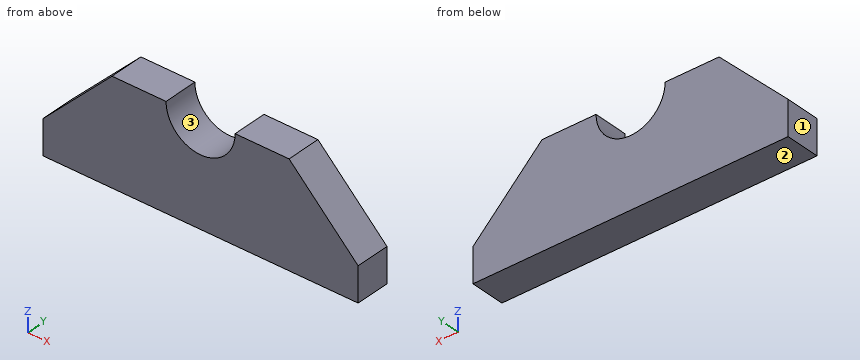
from build123d import *

# Parameters (mm, degrees)
F0_W     = 231.775
F0_H     = 25.4
F1_DEPTH = 76.2
F2_SIZE  = 50.8
F4_DEPTH = 25.4


with BuildPart() as f1:
    # F0 (on Top) → F1 (new body)
    with BuildSketch(Plane.XY):
        with Locations((-99.620111, 22.224578)):
            Rectangle(F0_W, F0_H)
    extrude(amount=F1_DEPTH)

    # F2
    f2_edges = [f1.edges().sort_by_distance(p)[0] for p in [
        (-215.507611, 22.224578, 76.2),
        (16.267389, 22.224578, 76.2),
    ]]
    chamfer(f2_edges, length=F2_SIZE)

    # F3 (on face) → F4 (cut)
    with BuildSketch(Plane.XZ.offset(-9.524578)):
        with BuildLine():
            Line((-125.020111, 76.2), (-74.220111, 76.2))
            ThreePointArc((-74.220111, 76.2), (-99.620111, 101.6), (-125.020111, 76.2))
        make_face()
        with BuildLine():
            ThreePointArc((-125.020111, 76.2), (-99.620111, 50.8), (-74.220111, 76.2))
            Line((-74.220111, 76.2), (-125.020111, 76.2))
        make_face()
    extrude(amount=-F4_DEPTH, mode=Mode.SUBTRACT)


solid = f1.part
CAD build for the part. Positions are in the model's coordinates, mm. Face numbers are marked on the shaded views. Coordinates: 2 decimals unless noted, no trailing zeros. Loops run counter-clockwise (first coordinate to the right, second up) from the corner with the lowest first, then second, coordinate; pieces in that order, holes last. Notation, with made-up numbers: (37, 25.5) - (77, 25.5) arc R22 ccw to (77, 51.5) - close; hole circle Ø3 at (46, 40.5). An arc over 180 degrees is marked (long way). Use one line per item in the form item = value. Start each with the question number.
1) Band-saw the part on B-B (z = 64). Give the cut face in (x, y).
2) Band-saw the part on A-A (y = 30.25). Give the cut face in (x, z), and give its area (3 significant figures).
3) Flat gauge pin, fed straight in: pin 1 (1 mm diameter, centred on x = -22.5, y = 22.5, fed in from +Z). Where does the tip first touch, or does it go through?
4) Drill centre lines: L1, parallel to Z at x = -206, y = 30; L2, parallel to X at y = 25.75, z = 68; L3, parallel to X at y = 19, z = 66.5 (3 decimals). Where is each one in solid material? Low to high. Write a range as from..to.
5) Two-plate mould, pull along X, no slides. Class the marked faces 1, 2 and 3: +X half, -X half, draft (parallel to the pull), parting line (faces both ways), or undercut.
6) Band-saw the part on C-C (z = 40). Give the cut face in (x, y), and give its area (3 significant figures).
7) Band-saw the part on D-D (x = -115). Give the cut face in (y, z), and give its area (3 significant figures).
Check values:
q1.outline = (-176.91, 9.52) - (-121.9, 9.52) - (-121.9, 34.92) - (-176.91, 34.92) - close; (-77.34, 9.52) - (-22.33, 9.52) - (-22.33, 34.92) - (-77.34, 34.92) - close
q2.outline = (-215.51, 0) - (16.27, 0) - (16.27, 25.4) - (-34.53, 76.2) - (-74.22, 76.2) arc R25.4 cw to (-125.02, 76.2) - (-164.71, 76.2) - (-215.51, 25.4) - close
q2.area = 14,100 mm2
q3.pin_1 = 64.67
q4.L1 = 0..34.91
q4.L2 = -172.91..-123.66, -75.58..-26.33
q4.L3 = -174.408..-123.095, -76.145..-24.833
q5.face_1 = -X half
q5.face_2 = draft
q5.face_3 = undercut
q6.outline = (-200.91, 9.52) - (1.67, 9.52) - (1.67, 34.92) - (-200.91, 34.92) - close
q6.area = 5,150 mm2
q7.outline = (9.52, 0) - (34.92, 0) - (34.92, 55.99) - (9.52, 55.99) - close
q7.area = 1,420 mm2
